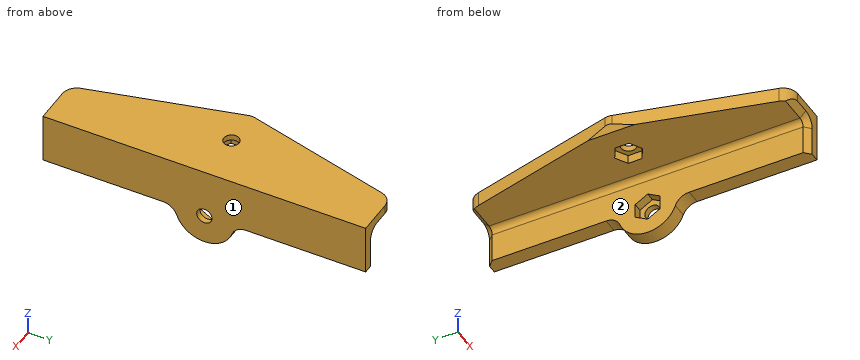
from build123d import *

# Parameters (mm, degrees)
BOSS_EXTRUDE1_DEPTH     = 30
CUT_EXTRUDE1_DEPTH      = 52.961524227
CUT_EXTRUDE1_DEPTH_BACK = 52.961524227
SKETCH2_R               = 2.6
CUT_EXTRUDE2_DEPTH      = 52.961524227
CUT_EXTRUDE2_DEPTH_BACK = 52.961524227
SKETCH3_R               = 2.6
CUT_EXTRUDE3_DEPTH      = 3
CUT_EXTRUDE4_DEPTH      = 3
BOSS_EXTRUDE4_DEPTH     = 40
BOSS_EXTRUDE5_START     = -30
BOSS_EXTRUDE5_DEPTH     = 40
FILLET2_R               = 5
FILLET3_R               = 2
CHAMFER2_SIZE           = 2
CUT_EXTRUDE7_DEPTH      = 81.156097709
CUT_EXTRUDE7_DEPTH_BACK = 81.156097709
FILLET4_R               = 5
CUT_EXTRUDE8_DEPTH      = 80.27168473
CUT_EXTRUDE8_DEPTH_BACK = 80.27168473
FILLET5_R               = 5


with BuildPart() as part:
    # Sketch1 → Boss-Extrude1 (new body)
    with BuildSketch(Plane(origin=(0, 0, 0), x_dir=(1, 0, 0), z_dir=(0, 1, 0))):
        Polygon((0, 0), (30, 0), (30, 30), (25, 30), (25, 5), (0, 5), align=None)
    extrude(amount=BOSS_EXTRUDE1_DEPTH)

    # Sketch2 → Cut-Extrude1 (cut, two sides: drawn at the far end of the back side and taken through both)
    with BuildSketch(Plane.XY.offset(-CUT_EXTRUDE1_DEPTH_BACK)):
        with Locations((13, 15)):
            Circle(SKETCH2_R)
    extrude(amount=CUT_EXTRUDE1_DEPTH + CUT_EXTRUDE1_DEPTH_BACK, mode=Mode.SUBTRACT)

    # Sketch3 → Cut-Extrude2 (cut, two sides: drawn at the far end of the back side and taken through both)
    with BuildSketch(Plane(origin=(30, 0, 0), x_dir=(0, 0, -1), z_dir=(1, 0, 0)).offset(-CUT_EXTRUDE2_DEPTH_BACK)):
        with Locations((17, 15)):
            Circle(SKETCH3_R)
    extrude(amount=CUT_EXTRUDE2_DEPTH + CUT_EXTRUDE2_DEPTH_BACK, mode=Mode.SUBTRACT)

    # Sketch4 → Cut-Extrude3 (cut)
    with BuildSketch(Plane.ZY.offset(-25)):
        Polygon((-21.907477288, 15), (-19.453738644, 10.75), (-14.546261356, 10.75), (-12.092522712, 15), (-14.546261356, 19.25), (-19.453738644, 19.25), align=None)
    extrude(amount=-CUT_EXTRUDE3_DEPTH, mode=Mode.SUBTRACT)

    # Sketch5 → Cut-Extrude4 (cut)
    with BuildSketch(Plane(origin=(0, 0, -5), x_dir=(-1, 0, 0), z_dir=(0, 0, -1))):
        Polygon((-17.1, 17.367136104), (-17.1, 12.632863896), (-13, 10.265727793), (-8.9, 12.632863896), (-8.9, 17.367136104), (-13, 19.734272207), align=None)
    extrude(amount=-CUT_EXTRUDE4_DEPTH, mode=Mode.SUBTRACT)

    # Sketch8 → Boss-Extrude4 (add)
    with BuildSketch(Plane(origin=(0, 30, 0), x_dir=(1, 0, 0), z_dir=(0, 1, 0))):
        Polygon((0, 5), (25, 5), (25, 30), (30, 30), (30, 0), (0, 0), align=None)
    extrude(amount=BOSS_EXTRUDE4_DEPTH)

    # Sketch8<2> → Boss-Extrude5 (add)
    with BuildSketch(Plane(origin=(0, 30, 0), x_dir=(1, 0, 0), z_dir=(0, 1, 0)).offset(BOSS_EXTRUDE5_START)):
        Polygon((0, 5), (25, 5), (25, 30), (30, 30), (30, 0), (0, 0), align=None)
    extrude(amount=-BOSS_EXTRUDE5_DEPTH)

    # Fillet2
    fillet2_edges = [part.edges().sort_by_distance(p)[0] for p in [
        (0, 70, -2.5),
        (27.5, 70, -30),
        (27.5, -40, -30),
        (0, -40, -2.5),
    ]]
    fillet(fillet2_edges, radius=FILLET2_R)

    # Fillet3
    fillet3_edges = [part.edges().sort_by_distance(p)[0] for p in [
        (25, 15, -5),
    ]]
    fillet(fillet3_edges, radius=FILLET3_R)

    # Chamfer2
    chamfer2_edges = [part.edges().sort_by_distance(p)[0] for p in [
        (25, 70, -16),
        (25, 15, -30),
        (25, -40, -16),
        (25, -38.535533906, -28.535533906),
        (25, 68.535533906, -28.535533906),
        (0, 15, -5),
        (1.464466094, -38.535533906, -5),
        (1.464466094, 68.535533906, -5),
        (14, 70, -5),
        (14, -40, -5),
        (24.414213562, -40, -5.585786438),
        (24.414213562, 70, -5.585786438),
    ]]
    chamfer(chamfer2_edges, length=CHAMFER2_SIZE)

    # Sketch11 → Cut-Extrude7 (cut, two sides: drawn at the far end of the back side and taken through both)
    with BuildSketch(Plane.ZY.offset(-25).offset(-CUT_EXTRUDE7_DEPTH_BACK)):
        with BuildLine():
            Line((-17, 25), (-17, 79.176495752))
            Line((-17, 79.176495752), (-82.490941739, 30.916627992))
            Line((-82.490941739, 30.916627992), (-67.497355256, -40.744999046))
            Line((-67.497355256, -40.744999046), (-17, -61.114612426))
            Line((-17, -61.114612426), (-17, 5))
            ThreePointArc((-17, 5), (-27, 15), (-17, 25))
        make_face()
    extrude(amount=CUT_EXTRUDE7_DEPTH + CUT_EXTRUDE7_DEPTH_BACK, mode=Mode.SUBTRACT)

    # Fillet4
    fillet4_edges = [part.edges().sort_by_distance(p)[0] for p in [
        (27.5, 25, -17),
        (27.5, 5, -17),
    ]]
    fillet(fillet4_edges, radius=FILLET4_R)

    # Sketch12 → Cut-Extrude8 (cut, two sides: drawn at the far end of the back side and taken through both)
    with BuildSketch(Plane(origin=(0, 0, -5), x_dir=(-1, 0, 0), z_dir=(0, 0, -1)).offset(-CUT_EXTRUDE8_DEPTH_BACK)):
        Polygon((-14, 70), (0, 15), (-14, -40), (29.605001417, -51.099454906), (59.954696555, 7.95039026), (29.605001417, 77.986583132), (-23, 76.936040239), align=None)
    extrude(amount=CUT_EXTRUDE8_DEPTH + CUT_EXTRUDE8_DEPTH_BACK, mode=Mode.SUBTRACT)

    # Fillet5
    fillet5_edges = [part.edges().sort_by_distance(p)[0] for p in [
        (14, -40, -1.5),
        (14, 70, -1.5),
        (0, 15, -1.5),
    ]]
    fillet(fillet5_edges, radius=FILLET5_R)


solid = part.part
The listing builds one solid part. Answer for the finished solid, in the listing's coordinates (mm). Face numbers are marked on the shaded views. A direction names the side the tool comes from. Coordinates: 2 decimals unless noted, no trailing zeros. Write each loop counter-clockwise with the first axis right and the second up, starting at its lowest first coordinate (ties: lowest second). Pieces come first, ordered by that corner, then holes. Notation, with made-up numbers: M 82,52.5 L 126,52.5 A17 ccw 126,58.5 Z; hole C -16.5,55.5 d2. An arc over 180 degrees is marked long. Write each question's results on one line, items separated by ' | '.
Item 1: Consider probe 1 along X at (y, z) = (15, -0.8); probe 2 along Z at (x, y) = (28.75, 15); probe 3 along Z at (x, y) = (8, 43). Determine where each line is inside the solid, lowest interval first. Write a range as [from, to].
Answer below:
probe 1: [0.16, 10.4], [15.6, 30] | probe 2: [-27, -19.6], [-14.4, 0] | probe 3: [-5, 0]
Item 2: The part is cut by section B-B on y = 44. Determine the outline of the cut face in (x, z).
Answer below:
outline: M 7.38,-5 L 23,-5 A2 cw 25,-7 L 25,-17 L 30,-17 L 30,0 L 7.38,0 Z
Item 3: The part is cut by section A-A on y = -13. Determine the outline of the cut face in (x, z).
Answer below:
outline: M 7.13,-5 L 23,-5 A2 cw 25,-7 L 25,-17 L 30,-17 L 30,0 L 7.13,0 Z
Item 4: Which of the six approach directions +Z, -Z, +X, -X, +Y, -Y give full straight-line access (tool end or side, diameter ignored) to the marked faces 1 and 2?
Answer below:
face 1: +Z, -Z, +X, +Y, -Y | face 2: -Z, -X, +Y, -Y
Item 5: Given P1, Ø5.5, axis at x = 28.5, y = -16.5, coming from the -Z side; P2, Ø1.5, axis at x = 26, z = -17, coming from the -Y side; P3, Ø6, axis at y = -9, z = -18, coming from the -X side, each flat-ended and moving along its own axis, determine where each tip first touches the part or whether it passes through.
Answer below:
P1: z = -17 | P2: y = -39.75 | P3: x = 25
